Build history of the part. All positions in model axes, mm. A direction names the side the tool comes from. Round coordinates to 2 decimals unless told otherwise and drop trailing zeros. Write each loop counter-clockwise with the first axis right and the second up, starting at its lowest first coordinate (ties: lowest second). Pieces come first, ordered by that corner, then holes. Notation, with made-up numbers: (-38, 52) -> (-1, 52) arc R38 cw to (-1, 91) -> close; hole circle Ø5 at (40, 42.5). An arc over 180 degrees is marked (long way). Answer in a Markdown table with one row per item. Add a question column.
from build123d import *

# Parameters (mm, degrees)
SKETCH1_R           = 4
BOSS_EXTRUDE1_DEPTH = 72
SKETCH2_W           = 8
SKETCH2_H           = 50
BOSS_EXTRUDE2_DEPTH = 70


with BuildPart() as part:
    # Sketch1 → Boss-Extrude1 (new body)
    with BuildSketch(Plane(origin=(0, 0, 0), x_dir=(1, 0, 0), z_dir=(0, 1, 0))):
        with Locations(Location((0, 0, 0), (0, 0, 270))):
            Circle(SKETCH1_R)
    extrude(amount=BOSS_EXTRUDE1_DEPTH)

    # Sketch2 → Boss-Extrude2 (add)
    with BuildSketch(Plane.XY):
        with Locations((0, 47)):
            Rectangle(SKETCH2_W, SKETCH2_H)
    extrude(amount=BOSS_EXTRUDE2_DEPTH)


solid = part.part
(1) Which spindle directions (+Z, -Z, +X, -X, +Y, -Y) get a long thin tool onto all of the face, cutting with end or side? Do faces 1 (the face through (0, 27, -4)), 2 (the face through (0, 0, 0)). Say none if no direction does.
(2) Probe line 1 along Z through (x, y) = (-0.25, 24); line 2 along Y through (x, z) = (0.5, 27.5); line 3 along Z through (x, y) = (0, 20.5). List the from-to ranges inside material, lowest first.
(3) Drop flat-ended pins along their axis: P1, Ø1, axis at x = -2, y = 9.5, coming from the +Z side; P2, Ø2, axis at x = -1.5, y = 12, coming from the -Z side. Give the stop position or say it passes through.
(4) Saw through at B-B (z = 24). List the corners of the cut face in (x, y), plus the area to 3 significant figures.
(5) Saw through at A-A (x = 0). List the corners of the cut face in (y, z), plus the area to 3 significant figures.
Answer sheet:
| question | item | result |
|---|---|---|
| 1 | face 1 | -Y |
| 1 | face 2 | +Z, -Z, +X, -X, -Y |
| 2 | line 1 | z = -3.99 to 70 |
| 2 | line 2 | y = 22 to 72 |
| 2 | line 3 | z = -4 to 4 |
| 3 | P1 | stops at z = 3.71 |
| 3 | P2 | stops at z = -3.97 |
| 4 | outline | (-4, 22) -> (4, 22) -> (4, 72) -> (-4, 72) -> close |
| 4 | area | 400 mm² |
| 5 | outline | (0, -4) -> (72, -4) -> (72, 70) -> (22, 70) -> (22, 4) -> (0, 4) -> close |
| 5 | area | 3,880 mm² |
